Model file for the job. Use its own axes, mm. Face numbers are marked on the shaded views. A direction names the side the tool comes from. Coordinates: 2 decimals unless noted, no trailing zeros. Order: outer loops, then holes, each group sorted by start corner. A loop starts at its lowest first (then second) coordinate and runs counter-clockwise, first axis right, second up. Notation, with made-up numbers: (12.5, -19) -> (56.5, -19) arc R25 ccw to (56.5, 8) -> close; hole circle Ø8 at (58.25, 76). An arc over 180 degrees is marked (long way). Return JSON: item names as keys, results as strings. Group by question number.
1) Cut at D-D (x = -22). Write the cut outline in (y, z), and give its area (3 significant figures).
2) Probe line 1 (Y direction, x = -34.5, z = 0.35); line 2 (Z direction, x = -26, y = 19); line 3 (X direction, y = 19.5, z = -3.5). List the from-to ranges inside material, lowest first.
3) Which spindle directions (+Z, -Z, +X, -X, +Y, -Y) get a long thin tool onto all of the face, cutting with end or side? Do the marked faces 1, 2, 3, 4 and 5. Say none if no direction does.
4) Cut at B-B (y = 2). Write the cut outline in (x, z).
5) Cut at A-A (x = -2). Write the cut outline in (y, z).
6) Flat gauge pins, fed straight in: pin 1 (5 mm diameter, centred on y = 16.5, z = -4, fed in from -X); pin 2 (3 mm diameter, centred on y = 26, z = -3.5, fed in from +X); pin 3 (1.1 mm diameter, centred on x = -17.5, y = 46.5, fed in from -Z); pin 4 (2 mm diameter, centred on x = -34.5, y = 2, fed in from -Z). Where does each tip first touch, or does it go through?
7) Cut at C-C (y = 38.5). Write the cut outline in (x, z).
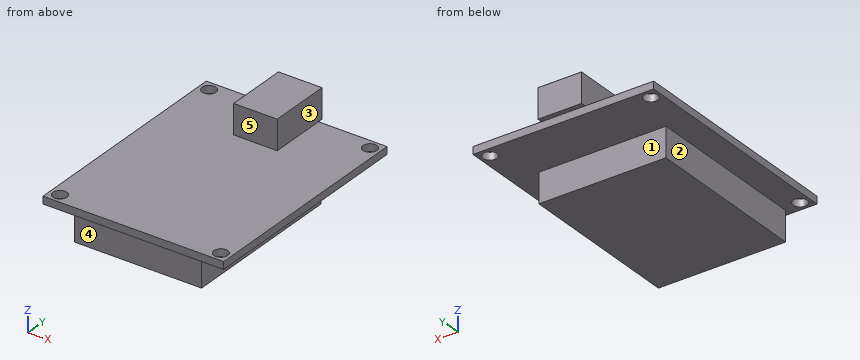
from build123d import *

# Parameters (mm, degrees)
F0_W     = 36.5
F0_H     = 46
F0_R     = 1.4
F1_DEPTH = 1.5
F2_W     = 8.8
F2_H     = 12.6
F3_DEPTH = 6
F4_W     = 25.7
F4_H     = 33.7
F5_DEPTH = 6


with BuildPart() as f1:
    # F0 (on Top) → F1 (new body)
    with BuildSketch(Plane.XY):
        with Locations((-18.25, 23)):
            Rectangle(F0_W, F0_H)
        with Locations((-34.5, 2)):
            Circle(F0_R, mode=Mode.SUBTRACT)
        with Locations((-2, 2)):
            Circle(F0_R, mode=Mode.SUBTRACT)
        with Locations((-34.5, 44)):
            Circle(F0_R, mode=Mode.SUBTRACT)
        with Locations((-2, 44)):
            Circle(F0_R, mode=Mode.SUBTRACT)
    extrude(amount=F1_DEPTH)

    # F2 (on face) → F3 (join)
    with BuildSketch(Plane.XY.offset(1.5)):
        with Locations((-18.25, 40.7)):
            Rectangle(F2_W, F2_H)
    extrude(amount=F3_DEPTH)

    # F4 (on face) → F5 (join)
    with BuildSketch(Plane(origin=(0, 0, 0), x_dir=(1, 0, 0), z_dir=(0, 0, -1))):
        with Locations((-18.25, -18.15)):
            Rectangle(F4_W, F4_H)
    extrude(amount=F5_DEPTH)


solid = f1.part
Answers below:
{
 "1": {"outline": "(0, 0) -> (1.3, 0) -> (1.3, -6) -> (35, -6) -> (35, 0) -> (46, 0) -> (46, 1.5) -> (47, 1.5) -> (47, 7.5) -> (34.4, 7.5) -> (34.4, 1.5) -> (0, 1.5) -> close", "area": "347 mm^2"},
 "2": {"line 1": "y = 0 to 0.6, 3.4 to 42.6, 45.4 to 46", "line 2": "z = -6 to 1.5", "line 3": "x = -31.1 to -5.4"},
 "3": {"face 1": "-Z, +X, -X, +Y", "face 2": "-Z, -X, +Y, -Y", "face 3": "+Z, +X, +Y, -Y", "face 4": "-Z, +X, -X, -Y", "face 5": "+Z, +X, -X, -Y"},
 "4": {"outline": "(-36.5, 0) -> (-35.9, 0) -> (-35.9, 1.5) -> (-36.5, 1.5) -> close; (-33.1, 0) -> (-31.1, 0) -> (-31.1, -6) -> (-5.4, -6) -> (-5.4, 0) -> (-3.4, 0) -> (-3.4, 1.5) -> (-33.1, 1.5) -> close; (-0.6, 0) -> (0, 0) -> (0, 1.5) -> (-0.6, 1.5) -> close"},
 "5": {"outline": "(0, 0) -> (0.6, 0) -> (0.6, 1.5) -> (0, 1.5) -> close; (3.4, 0) -> (42.6, 0) -> (42.6, 1.5) -> (3.4, 1.5) -> close; (45.4, 0) -> (46, 0) -> (46, 1.5) -> (45.4, 1.5) -> close"},
 "6": {"pin 1": "stops at x = -31.1", "pin 2": "stops at x = -5.4", "pin 3": "stops at z = 0", "pin 4": "passes through"},
 "7": {"outline": "(-36.5, 0) -> (0, 0) -> (0, 1.5) -> (-13.85, 1.5) -> (-13.85, 7.5) -> (-22.65, 7.5) -> (-22.65, 1.5) -> (-36.5, 1.5) -> close"}
}
